Job drawing, mm, ordinate dimensions from the low corner. One solid piece. A direction names the side the tool comes from. Coordinates: 2 decimals unless noted, no trailing zeros. Loops run counter-clockwise (first coordinate to the right, second up) from the corner with the lowest first, then second, coordinate; pieces in that order, holes last. Notation, with made-up numbers: (51.25, 51) - (110.25, 51) arc R28 cw to (110.25, 73) - close; hole circle Ø2 at (-8.5, -32). An arc over 180 degrees is marked (long way). Use a Markdown table: item, result. Add a question column.
1) Band-saw the part on D-D (y = 1.75). Give the cut face in (x, z).
2) Probe probe 1 along X at (y, z) = (6.5, 4.4) (1 decimal); probe 2 along X at (y, z) = (5.25, 2.4) (1 decimal); probe 3 along Y at (x, z) = (13.5, 1.85). List the from-to ranges inside material, lowest first. Write a range as [from, to].
3) Drop flat-ended pins along their axis: P1, Ø3, axis at y = 6, z = 2, coming from the +X side (1 decimal); P2, Ø2, axis at x = 16.5, z = 1.5, coming from the -Y side; P3, Ø3, axis at y = 6, z = 3, coming from the -X side (1 decimal). Give the stop position or say it passes through.
4) Band-saw the part on C-C (x = 37). Give the cut face in (y, z).
5) Pull direction X, two halves, no side cores. Call the marked faces 1, 2 and 3: +X half, -X half, draft (parallel to the pull), parting line (faces both ways), or undercut.
6) Tool access for the marked faces 4 and 5: list every direction of +Z, -Z, +X, -X, +Y, -Y with a clear straight run to the whole face (end or side of a thin tool).
7) Band-saw the part on B-B (y = 11.75). Give the cut face in (x, z).
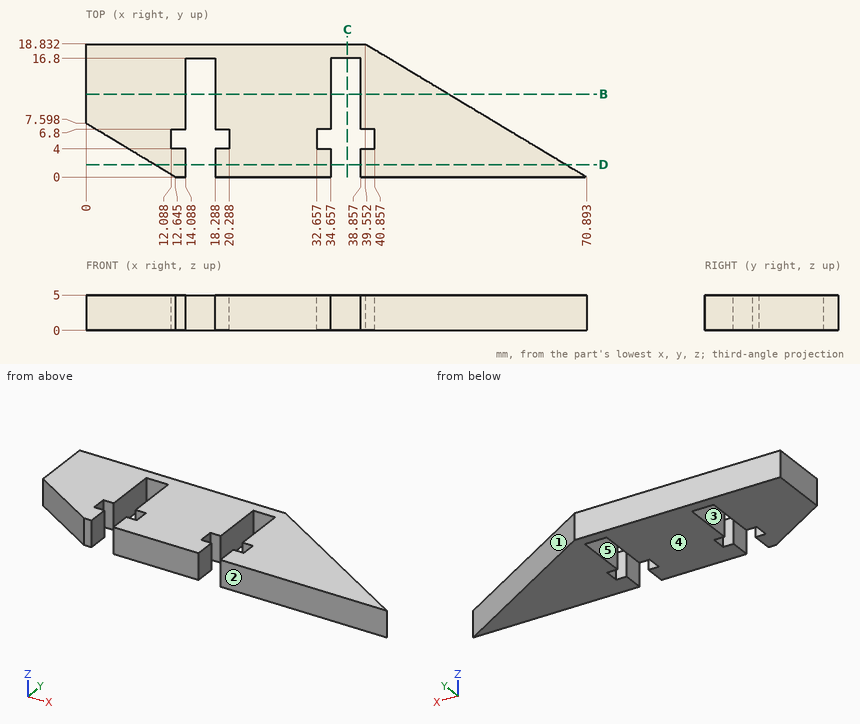
Answer block:
| question | item | result |
|---|---|---|
| 1 | outline | (9.73, 0) - (14.09, 0) - (14.09, 5) - (9.73, 5) - close; (18.29, 0) - (34.66, 0) - (34.66, 5) - (18.29, 5) - close; (38.86, 0) - (67.98, 0) - (67.98, 5) - (38.86, 5) - close |
| 2 | probe 1 | [1.8, 12.1], [20.3, 32.7], [40.9, 60.1] |
| 2 | probe 2 | [3.9, 12.1], [20.3, 32.7], [40.9, 62.2] |
| 2 | probe 3 | [0, 4], [6.8, 18.83] |
| 3 | P1 | x = 63.4 |
| 3 | P2 | y = 16.8 |
| 3 | P3 | x = 0.2 |
| 4 | outline | (16.8, 0) - (18.83, 0) - (18.83, 5) - (16.8, 5) - close |
| 5 | face 1 | +X half |
| 5 | face 2 | draft |
| 5 | face 3 | undercut |
| 6 | face 4 | -Z, +X, -X, +Y, -Y |
| 6 | face 5 | +Z, -Z, -Y |
| 7 | outline | (0, 0) - (14.09, 0) - (14.09, 5) - (0, 5) - close; (18.29, 0) - (34.66, 0) - (34.66, 5) - (18.29, 5) - close; (38.86, 0) - (51.34, 0) - (51.34, 5) - (38.86, 5) - close |
